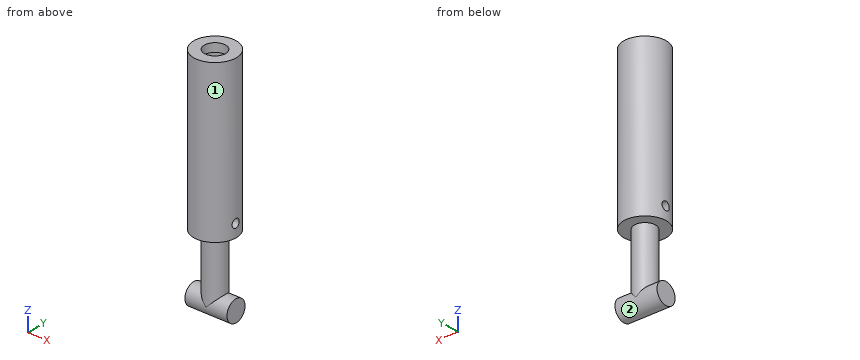
from build123d import *

# Parameters (mm, degrees)
SKETCH1_R                = 5
BOSS_EXTRUDE1_DEPTH      = 37
SKETCH2_R                = 2.5
CUT_EXTRUDE1_DEPTH       = 2
SKETCH3_R                = 3
CUT_EXTRUDE2_DEPTH       = 33
CUT_EXTRUDE3_START       = -5.000000101
CUT_EXTRUDE3_OUTLINE_R   = 1
CUT_EXTRUDE3_DEPTH       = 10.000000201
SKETCH4_R                = 2.5
BOSS_EXTRUDE2_DEPTH      = 15
BOSS_EXTRUDE3_DEPTH      = 5
BOSS_EXTRUDE3_DEPTH_BACK = 5
SKETCH5_R                = 2.5


# Read off the part's stored shape, not the designer's step: Cut-Extrude3
with BuildPart() as part:
    # Sketch1 → Boss-Extrude1 (new body)
    with BuildSketch(Plane.XY):
        Circle(SKETCH1_R)
    extrude(amount=BOSS_EXTRUDE1_DEPTH)

    # Sketch2 → Cut-Extrude1 (cut)
    with BuildSketch(Plane.XY.offset(37)):
        Circle(SKETCH2_R)
    extrude(amount=-CUT_EXTRUDE1_DEPTH, mode=Mode.SUBTRACT)

    # Sketch3 → Cut-Extrude2 (cut)
    with BuildSketch(Plane.XY.offset(35)):
        Circle(SKETCH3_R)
    extrude(amount=-CUT_EXTRUDE2_DEPTH, mode=Mode.SUBTRACT)

    # Cut-Extrude3 outline → Cut-Extrude3 (cut)
    with BuildSketch(Plane.YZ.offset(CUT_EXTRUDE3_START)):
        with Locations((0, 3)):
            Circle(CUT_EXTRUDE3_OUTLINE_R)
    extrude(amount=CUT_EXTRUDE3_DEPTH, mode=Mode.SUBTRACT)

    # Sketch4 → Boss-Extrude2 (add)
    with BuildSketch(Plane(origin=(0, 0, 0), x_dir=(-1, 0, 0), z_dir=(0, 0, -1))):
        with Locations(Location((0, 0, 0), (0, 0, 180))):
            Circle(SKETCH4_R)
    extrude(amount=BOSS_EXTRUDE2_DEPTH)

    # Sketch5 → Boss-Extrude3 (add, two sides: drawn at the far end of the back side and taken through both)
    with BuildSketch(Plane(origin=(0, 0, 0), x_dir=(0, 0, -1), z_dir=(1, 0, 0)).offset(-BOSS_EXTRUDE3_DEPTH_BACK)):
        with Locations((15, 0)):
            Circle(SKETCH5_R)
    extrude(amount=BOSS_EXTRUDE3_DEPTH + BOSS_EXTRUDE3_DEPTH_BACK)


solid = part.part
Build history of the part. All positions in model axes, mm. Face numbers are marked on the shaded views. A direction names the side the tool comes from. Round coordinates to 2 decimals unless told otherwise and drop trailing zeros. Write each loop counter-clockwise with the first axis right and the second up, starting at its lowest first coordinate (ties: lowest second). Pieces come first, ordered by that corner, then holes. Notation, with made-up numbers: (60, 77) -> (114, 77) arc R26 ccw to (114, 114) -> close; hole circle Ø4 at (78.5, -15). An arc over 180 degrees is marked (long way). Use one line per item in the form item = value.
Q1. Tool access for the marked faces 1 and 2: list every direction of +Z, -Z, +X, -X, +Y, -Y with a clear straight run to the whole face (end or side of a thin tool).
Conclusion:
face_1 = +Z
face_2 = none
Q2. Band-saw the part on C-C, the plane x = -3.5. Write the cut outline in (y, z), then the cut area to 3 significant figures.
Conclusion:
outline = (-3.57, 0) -> (3.57, 0) -> (3.57, 37) -> (-3.57, 37) -> close; circle Ø5 at (0, -15); hole circle Ø2 at (0, 3)
area = 281 mm²
Q3. Band-saw the part on B-B, the plane z = 3. Write the cut outline in (x, y), then the cut area to 3 significant figures.
Conclusion:
outline = (-4.9, -1) arc R5 ccw to (4.9, -1) -> (2.83, -1) arc R3 cw to (-2.83, -1) -> close; (-4.9, 1) -> (-2.83, 1) arc R3 cw to (2.83, 1) -> (4.9, 1) arc R5 ccw to start
area = 42.2 mm²
Q4. Drill centre lines: L1, parallel to Y at x = 0, z = 15.5; L2, parallel to Z at x = 2.75, y = 0.75; L3, parallel to Z at x = 3.75, y = 0.25. Where is each one in solid material? Low to high.
Conclusion:
L1 = -5 to -3, 3 to 5
L2 = -17.38 to -12.62, 0 to 2, 35 to 37
L3 = -17.49 to -12.51, 0 to 2.03, 3.97 to 37
Q5. Band-saw the part on A-A, the plane x = 0. Write the cut outline in (y, z), then the cut area to 3 significant figures.
Conclusion:
outline = (-5, 0) -> (-2.5, 0) -> (-2.5, -15) arc R2.5 ccw to (2.5, -15) -> (2.5, 0) -> (5, 0) -> (5, 37) -> (2.5, 37) -> (2.5, 35) -> (3, 35) -> (3, 2) -> (-3, 2) -> (-3, 35) -> (-2.5, 35) -> (-2.5, 37) -> (-5, 37) -> close
area = 247 mm²
Q6. Band-saw the part on D-D, the plane y = -4. Write the cut outline in (x, z), then the cut area to 3 significant figures.
Conclusion:
outline = (-3, 0) -> (3, 0) -> (3, 37) -> (-3, 37) -> close
area = 222 mm²
Q7. Drop flat-ended pins along their axis: P1, Ø2, axis at x = 3, z = 23.5, coming from the -Y side; P2, Ø5, axis at x = -1, z = -9.5, coming from the +Y side; P3, Ø4, axis at y = -0.5, z = -8.5, coming from the +X side. Give the stop position or say it passes through.
Conclusion:
P1 = -4.58
P2 = 2.5
P3 = 2.5
